Source: CAD feature listing. Evaluate the final solid. Frame: model axes, mm. Give positions to 0.01 mm unless a question says otherwise; leave off trailing zeros. Write each loop counter-clockwise with the first axis right and the second up, starting at its lowest first coordinate (ties: lowest second). Pieces come first, ordered by that corner, then holes. Notation, with made-up numbers: (56.25, 67) -> (67.25, 67) arc R31 ccw to (67.25, 102) -> close; hole circle Ø9 at (-30.5, 23.25). An arc over 180 degrees is marked (long way). Answer as a JSON object with one key per item and string values. Group by question number.
Item 1: Ray query, probe 1 along Z at (x, y) = (1, 0.9); probe 2 along Z at (x, y) = (0.25, 0.3); probe 3 along Z at (x, y) = (-11.75, 0.35). Return the intervals inside material, ascending. Write a range as from..to.
Item 2: First-contact query: pin 1 Ø1 at (y, z) = (0.5, -26) entering from -X; pin 2 Ø0.6 at (y, z) = (1, 8) entering from +X. Flat tips, straight axial feed; report the tip coordinate or a pass-through.
Item 3: Section query C-C on x = -8.5. Return the cut outline in (y, z), plus the area to 3 significant figures.
Item 4: Section query A-A on y = 1.1. Return the cut outline in (x, z), plus the area to 3 significant figures.
Item 5: Section query D-D on z = -15. Return the cut outline in (x, y).
Item 6: Section query B-B on z = 10. Return the cut outline in (x, y), plus the area to 3 significant figures.
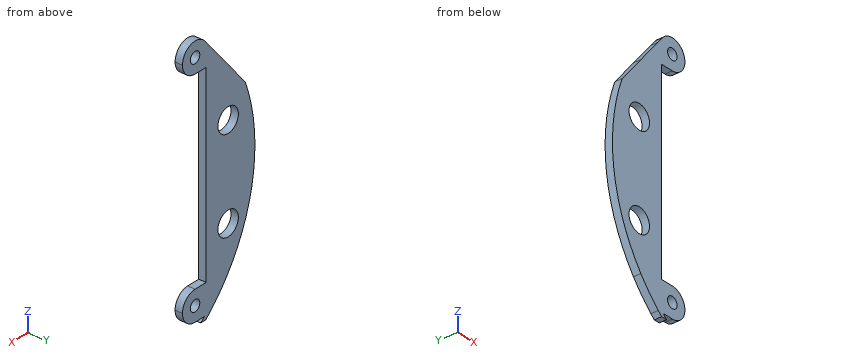
from build123d import *

# Parameters (mm, degrees)
SKETCH_1_W          = 20
SKETCH_1_H          = 70
SKETCH_1_R          = 1.5
SKETCH_1_W_2        = 6
SKETCH_1_H_2        = 52
EXTRUDE_1_DEPTH     = 2
SKETCH_2_W          = 0.5
SKETCH_2_H          = 26
CUT_EXTRUDE_1_DEPTH = 37.455452267
EXTRUDE_3_DEPTH     = 2
SKETCH_4_R          = 3.25
CUT_EXTRUDE_2_DEPTH = 40.874804075


with BuildPart() as part:
    # Эскиз1 → Бобышка-Вытянуть1 (new body)
    with BuildSketch(Plane(origin=(0, 0, 0), x_dir=(1, 0, 0), z_dir=(0, 1, 0))):
        Rectangle(SKETCH_1_W, SKETCH_1_H)
        with Locations(Location((0, 30, 0), (0, 0, 270))):
            Circle(SKETCH_1_R, mode=Mode.SUBTRACT)
        with Locations(Location((0, -30, 0), (0, 0, 270))):
            Circle(SKETCH_1_R, mode=Mode.SUBTRACT)
        Rectangle(SKETCH_1_W_2, SKETCH_1_H_2, mode=Mode.SUBTRACT)
    extrude(amount=EXTRUDE_1_DEPTH)

    # Эскиз2 → Вырез-Вытянуть1 (cut, through all)
    with BuildSketch(Plane(origin=(0, 2, 0), x_dir=(1, 0, 0), z_dir=(0, 1, 0))):
        with Locations((-3.25, -13)):
            Rectangle(SKETCH_2_W, SKETCH_2_H)
        with Locations((-3.25, 13)):
            Rectangle(SKETCH_2_W, SKETCH_2_H)
        with BuildLine():
            ThreePointArc((4, 30), (2.828427125, 27.171572875), (0, 26))
            Line((0, 26), (3, 26))
            Line((3, 26), (3, 0))
            Line((3, 0), (10, 0))
            Line((10, 0), (10, 35))
            Line((10, 35), (-1.801814511, 35))
            ThreePointArc((-1.801814511, 35), (-2.371833534, 34.50465844), (-2.933620688, 34))
            Line((-2.933620688, 34), (0, 34))
            ThreePointArc((0, 34), (2.828427125, 32.828427125), (4, 30))
        make_face()
        with BuildLine():
            ThreePointArc((-10, 27.658633372), (-7.367393186, 30.953957731), (-4.449961479, 34))
            ThreePointArc((-4.449961479, 34), (-3.913284985, 34.504235123), (-3.368774283, 35))
            Line((-3.368774283, 35), (-10, 35))
            Line((-10, 35), (-10, 27.658633372))
        make_face()
        with BuildLine():
            Line((10, 0), (3, 0))
            Line((3, 0), (3, -26))
            Line((3, -26), (0, -26))
            ThreePointArc((0, -26), (2.828427125, -27.171572875), (4, -30))
            ThreePointArc((4, -30), (1.336481718, -33.770121565), (-3.106908308, -32.519349274))
            Line((-3.106908308, -32.519349274), (-4.5, -30.80136273))
            Line((-4.5, -30.80136273), (-4.5, -32.5))
            ThreePointArc((-4.5, -32.5), (-3.175976694, -33.777056798), (-1.801814511, -35))
            Line((-1.801814511, -35), (10, -35))
            Line((10, -35), (10, 0))
        make_face()
        with BuildLine():
            Line((-4.5, -32.5), (-4.5, -30.80136273))
            Line((-4.5, -30.80136273), (-10, -24.018660595))
            Line((-10, -24.018660595), (-10, -35))
            Line((-10, -35), (-1.801814511, -35))
            ThreePointArc((-1.801814511, -35), (-3.175976694, -33.777056798), (-4.5, -32.5))
        make_face()
    extrude(amount=-CUT_EXTRUDE_1_DEPTH, mode=Mode.SUBTRACT)

    # Эскиз3 → Бобышка-Вытянуть3 (add)
    with BuildSketch(Plane(origin=(0, 2, 0), x_dir=(1, 0, 0), z_dir=(0, 1, 0))):
        with BuildLine():
            Line((-15.931618932, -16.703677979), (-10, -24.018660595))
            Line((-10, -24.018660595), (-10, 27.658633372))
            ThreePointArc((-10, 27.658633372), (-18.585418451, 6.228867289), (-15.931618932, -16.703677979))
        make_face()
    extrude(amount=-EXTRUDE_3_DEPTH)

    # Эскиз4 → Вырез-Вытянуть2 (cut, through all)
    with BuildSketch(Plane(origin=(0, 2, 0), x_dir=(1, 0, 0), z_dir=(0, 1, 0))):
        with Locations(Location((-10.5, 15, 0), (0, 0, 270))):
            Circle(SKETCH_4_R)
        with Locations(Location((-10.5, -10, 0), (0, 0, 270))):
            Circle(SKETCH_4_R)
    extrude(amount=-CUT_EXTRUDE_2_DEPTH, mode=Mode.SUBTRACT)


solid = part.part
Worked answers:
{
 "1": {"probe 1": "-33.87..-31.12, -28.88..-26.13, 26.13..28.88, 31.12..33.87", "probe 2": "-33.99..-31.48, -28.52..-26.01, 26.01..28.52, 31.48..33.99", "probe 3": "-25.08..-18, -12..7, 13..21.86"},
 "2": {"pin 1": "x = -11.48", "pin 2": "x = -3.5"},
 "3": {"outline": "(0, -29.61) -> (2, -29.61) -> (2, -17.56) -> (0, -17.56) -> close; (0, -12.44) -> (2, -12.44) -> (2, 7.44) -> (0, 7.44) -> close; (0, 12.56) -> (2, 12.56) -> (2, 25.87) -> (0, 25.87) -> close", "area": "90.5 mm^2"},
 "4": {"outline": "(-15.93, 16.7) arc R47 ccw to (-4.45, -34) arc R47 ccw to (-3.37, -35) -> (-1.8, -35) arc R45.87 cw to (-2.93, -34) -> (0, -34) arc R4 ccw to (0, -26) -> (-3.5, -26) -> (-3.5, 26) -> (0, 26) arc R4 ccw (long way) to (-3.11, 32.52) -> close; hole circle Ø6.5 at (-10.5, -15); hole circle Ø6.5 at (-10.5, 10); hole circle Ø3 at (0, -30); hole circle Ø3 at (0, 30)", "area": "736 mm^2"},
 "5": {"outline": "(-16.54, 0) -> (-13.75, 0) -> (-13.75, 2) -> (-16.54, 2) -> close; (-7.25, 0) -> (-3.5, 0) -> (-3.5, 2) -> (-7.25, 2) -> close"},
 "6": {"outline": "(-17.92, 0) -> (-13.75, 0) -> (-13.75, 2) -> (-17.92, 2) -> close; (-7.25, 0) -> (-3.5, 0) -> (-3.5, 2) -> (-7.25, 2) -> close", "area": "15.8 mm^2"}
}
